Geometry: final body of the model. Coordinates: model frame, mm. A direction names the side the tool comes from. Give positions to 0.01 mm unless a question says otherwise; leave off trailing zeros. Loops run counter-clockwise (first coordinate to the right, second up) from the corner with the lowest first, then second, coordinate; pieces in that order, holes last.
from build123d import *

# Parameters (mm, degrees)
ESQUISSE1_W                          = 200
ESQUISSE1_H                          = 300
BOSS_EXTRU_1_DEPTH                   = 80
COQUE1_T                             = -4
ESQUISSE3_W                          = 196.2
ESQUISSE3_H                          = 296.2
ENL_V_MAT_EXTRU_2_DEPTH              = 4.1
ESQUISSE4_R                          = 9
BOSS_EXTRU_2_DEPTH                   = 67.9
ESQUISSE5_R                          = 2.5
ENL_V_MAT_EXTRU_3_DEPTH              = 30
ESQUISSE4_4_R                        = 9
BOSS_EXTRU_3_DEPTH                   = 15
ESQUISSE6_R                          = 2.5
ENL_V_MAT_EXTRU_6_DEPTH              = 10
ESQUISSE8_R                          = 9
BOSS_EXTRU_5_DEPTH                   = 68
ESQUISSE9_R                          = 2.5
ENL_V_MAT_EXTRU_8_DEPTH              = 30
ESQUISSE10_W                         = 1.9
ESQUISSE10_H                         = 2.840533171
BOSS_EXTRU_6_DEPTH                   = 10
R_P_TITION_LIN_AIRE1_COUNT           = 2
R_P_TITION_LIN_AIRE1_PITCH           = 198.1
R_P_TITION_LIN_AIRE2_COUNT           = 3
R_P_TITION_LIN_AIRE2_PITCH           = 130
R_P_TITION_LIN_AIRE2_COPY_1_SKETCH_W = 1.9
R_P_TITION_LIN_AIRE2_COPY_1_SKETCH_H = 2.840533171
R_P_TITION_LIN_AIRE2_COPY_1_DEPTH    = 10
R_P_TITION_LIN_AIRE2_COPY_2_SKETCH_W = 1.9
R_P_TITION_LIN_AIRE2_COPY_2_SKETCH_H = 2.840533171
R_P_TITION_LIN_AIRE2_COPY_2_DEPTH    = 10


with BuildPart() as part:
    # Esquisse1 → Boss.-Extru.1 (new body)
    with BuildSketch(Plane.XY):
        with Locations((43.373964051, -118.711656442)):
            Rectangle(ESQUISSE1_W, ESQUISSE1_H)
    extrude(amount=BOSS_EXTRU_1_DEPTH)

    # Coque1
    coque1_openings = [part.faces().sort_by_distance(p)[0] for p in [
        (43.373964051, -118.711656442, 0),
    ]]
    offset(amount=COQUE1_T, openings=coque1_openings, kind=Kind.INTERSECTION)

    # Esquisse3 → Enl_v. mat.-Extru.2 (cut)
    with BuildSketch(Plane(origin=(0, 0, 0), x_dir=(-1, 0, 0), z_dir=(0, 0, -1))):
        with Locations((-43.373964051, -118.711656442)):
            Rectangle(ESQUISSE3_W, ESQUISSE3_H)
    extrude(amount=-ENL_V_MAT_EXTRU_2_DEPTH, mode=Mode.SUBTRACT)

    # Esquisse4 → Boss.-Extru.2 (add)
    with BuildSketch(Plane(origin=(0, 0, 76), x_dir=(-1, 0, 0), z_dir=(0, 0, -1))):
        with Locations((-119.373964051, 7.288343558)):
            Circle(ESQUISSE4_R)
    extrude(amount=BOSS_EXTRU_2_DEPTH)

    # Esquisse5 → Enl_v. mat.-Extru.3 (cut)
    with BuildSketch(Plane(origin=(0, 0, 8.1), x_dir=(-1, 0, 0), z_dir=(0, 0, -1))):
        with Locations((-119.373964051, 7.288343558)):
            Circle(ESQUISSE5_R)
    extrude(amount=-ENL_V_MAT_EXTRU_3_DEPTH, mode=Mode.SUBTRACT)

    # Esquisse4_4 → Boss.-Extru.3 (add)
    with BuildSketch(Plane(origin=(0, 0, 76), x_dir=(-1, 0, 0), z_dir=(0, 0, -1))):
        with BuildLine():
            Line((-101.873964051, -42.711656442), (-101.873964051, -51.711656442))
            Line((-101.873964051, -51.711656442), (-110.873964051, -51.711656442))
            ThreePointArc((-110.873964051, -51.711656442), (-101.873964051, -60.711656442), (-92.873964051, -51.711656442))
            ThreePointArc((-92.873964051, -51.711656442), (-95.510003021, -45.347695411), (-101.873964051, -42.711656442))
        make_face()
        with BuildLine():
            Line((-110.873964051, -51.711656442), (-101.873964051, -51.711656442))
            Line((-101.873964051, -51.711656442), (-101.873964051, -42.711656442))
            ThreePointArc((-101.873964051, -42.711656442), (-108.237925082, -45.347695411), (-110.873964051, -51.711656442))
        make_face()
        with BuildLine():
            Line((-101.873964051, -42.711656442), (-101.873964051, -51.711656442))
            Line((-101.873964051, -51.711656442), (-110.873964051, -51.711656442))
            ThreePointArc((-110.873964051, -51.711656442), (-101.873964051, -60.711656442), (-92.873964051, -51.711656442))
            ThreePointArc((-92.873964051, -51.711656442), (-95.510003021, -45.347695411), (-101.873964051, -42.711656442))
        make_face()
        with BuildLine():
            Line((-110.873964051, -51.711656442), (-101.873964051, -51.711656442))
            Line((-101.873964051, -51.711656442), (-101.873964051, -42.711656442))
            ThreePointArc((-101.873964051, -42.711656442), (-108.237925082, -45.347695411), (-110.873964051, -51.711656442))
        make_face()
        with BuildLine():
            Line((15.126035949, -194.711656442), (15.126035949, -185.711656442))
            Line((15.126035949, -185.711656442), (24.126035949, -185.711656442))
            ThreePointArc((24.126035949, -185.711656442), (8.762074918, -179.347695411), (15.126035949, -194.711656442))
        make_face()
        with BuildLine():
            Line((24.126035949, -185.711656442), (15.126035949, -185.711656442))
            Line((15.126035949, -185.711656442), (15.126035949, -194.711656442))
            ThreePointArc((15.126035949, -194.711656442), (21.489996979, -192.075617472), (24.126035949, -185.711656442))
        make_face()
        with BuildLine():
            Line((15.126035949, -194.711656442), (15.126035949, -185.711656442))
            Line((15.126035949, -185.711656442), (24.126035949, -185.711656442))
            ThreePointArc((24.126035949, -185.711656442), (8.762074918, -179.347695411), (15.126035949, -194.711656442))
        make_face()
        with BuildLine():
            Line((24.126035949, -185.711656442), (15.126035949, -185.711656442))
            Line((15.126035949, -185.711656442), (15.126035949, -194.711656442))
            ThreePointArc((15.126035949, -194.711656442), (21.489996979, -192.075617472), (24.126035949, -185.711656442))
        make_face()
        with Locations((15.126035949, -51.711656442)):
            Circle(ESQUISSE4_4_R)
        with Locations((-101.873964051, -185.711656442)):
            Circle(ESQUISSE4_4_R)
    extrude(amount=BOSS_EXTRU_3_DEPTH)

    # Esquisse6 → Enl_v. mat.-Extru.6 (cut)
    with BuildSketch(Plane(origin=(0, 0, 61), x_dir=(-1, 0, 0), z_dir=(0, 0, -1))):
        with Locations((-101.873964051, -51.711656442)):
            Circle(ESQUISSE6_R)
        with Locations((15.126035949, -51.711656442)):
            Circle(ESQUISSE6_R)
        with Locations((-101.873964051, -185.711656442)):
            Circle(ESQUISSE6_R)
        with Locations((15.126035949, -185.711656442)):
            Circle(ESQUISSE6_R)
    extrude(amount=-ENL_V_MAT_EXTRU_6_DEPTH, mode=Mode.SUBTRACT)

    # Esquisse8 → Boss.-Extru.5 (add)
    with BuildSketch(Plane(origin=(0, 0, 76), x_dir=(-1, 0, 0), z_dir=(0, 0, -1))):
        with BuildLine():
            Line((32.626035949, 16.288343558), (32.626035949, 7.288343558))
            Line((32.626035949, 7.288343558), (41.626035949, 7.288343558))
            ThreePointArc((41.626035949, 7.288343558), (38.989996979, 13.652304589), (32.626035949, 16.288343558))
        make_face()
        with BuildLine():
            Line((41.626035949, 7.288343558), (32.626035949, 7.288343558))
            Line((32.626035949, 7.288343558), (32.626035949, 16.288343558))
            ThreePointArc((32.626035949, 16.288343558), (26.262074918, 0.924382528), (41.626035949, 7.288343558))
        make_face()
        with BuildLine():
            Line((32.626035949, 16.288343558), (32.626035949, 7.288343558))
            Line((32.626035949, 7.288343558), (41.626035949, 7.288343558))
            ThreePointArc((41.626035949, 7.288343558), (38.989996979, 13.652304589), (32.626035949, 16.288343558))
        make_face()
        with BuildLine():
            Line((41.626035949, 7.288343558), (32.626035949, 7.288343558))
            Line((32.626035949, 7.288343558), (32.626035949, 16.288343558))
            ThreePointArc((32.626035949, 16.288343558), (26.262074918, 0.924382528), (41.626035949, 7.288343558))
        make_face()
        with BuildLine():
            Line((32.626035949, -253.711656442), (32.626035949, -244.711656442))
            Line((32.626035949, -244.711656442), (41.626035949, -244.711656442))
            ThreePointArc((41.626035949, -244.711656442), (26.262074918, -238.347695411), (32.626035949, -253.711656442))
        make_face()
        with BuildLine():
            Line((41.626035949, -244.711656442), (32.626035949, -244.711656442))
            Line((32.626035949, -244.711656442), (32.626035949, -253.711656442))
            ThreePointArc((32.626035949, -253.711656442), (38.989996979, -251.075617472), (41.626035949, -244.711656442))
        make_face()
        with BuildLine():
            Line((32.626035949, -253.711656442), (32.626035949, -244.711656442))
            Line((32.626035949, -244.711656442), (41.626035949, -244.711656442))
            ThreePointArc((41.626035949, -244.711656442), (26.262074918, -238.347695411), (32.626035949, -253.711656442))
        make_face()
        with BuildLine():
            Line((41.626035949, -244.711656442), (32.626035949, -244.711656442))
            Line((32.626035949, -244.711656442), (32.626035949, -253.711656442))
            ThreePointArc((32.626035949, -253.711656442), (38.989996979, -251.075617472), (41.626035949, -244.711656442))
        make_face()
        with Locations((-119.373964051, -244.711656442)):
            Circle(ESQUISSE8_R)
    extrude(amount=BOSS_EXTRU_5_DEPTH)

    # Esquisse9 → Enl_v. mat.-Extru.8 (cut)
    with BuildSketch(Plane(origin=(0, 0, 8), x_dir=(-1, 0, 0), z_dir=(0, 0, -1))):
        with Locations((32.626035949, 7.288343558)):
            Circle(ESQUISSE9_R)
        with Locations((32.626035949, -244.711656442)):
            Circle(ESQUISSE9_R)
        with Locations((-119.373964051, -244.711656442)):
            Circle(ESQUISSE9_R)
    extrude(amount=-ENL_V_MAT_EXTRU_8_DEPTH, mode=Mode.SUBTRACT)

    # Esquisse10 → Boss.-Extru.6 (add)
    with BuildSketch(Plane(origin=(0, 0, 0), x_dir=(-1, 0, 0), z_dir=(0, 0, -1))):
        with Locations((-142.423964051, -249.983146828)):
            Rectangle(ESQUISSE10_W, ESQUISSE10_H)
    boss_extru_6 = extrude(amount=BOSS_EXTRU_6_DEPTH)

    # R_p_tition lin_aire1: Boss.-Extru.6 ×2
    with Locations(*[(-i * R_P_TITION_LIN_AIRE1_PITCH, 0, 0) for i in range(1, R_P_TITION_LIN_AIRE1_COUNT)]):
        add(boss_extru_6)

    # R_p_tition lin_aire2: Boss.-Extru.6 ×3
    with Locations(*[(0, i * R_P_TITION_LIN_AIRE2_PITCH, 0) for i in range(1, R_P_TITION_LIN_AIRE2_COUNT)]):
        add(boss_extru_6)

    # R_p_tition lin_aire2 copy 1 sketch → R_p_tition lin_aire2 copy 1 (add)
    with BuildSketch(Plane(origin=(-198.1, 130, 0), x_dir=(-1, 0, 0), z_dir=(0, 0, -1))):
        with Locations((-142.423964051, -249.983146828)):
            Rectangle(R_P_TITION_LIN_AIRE2_COPY_1_SKETCH_W, R_P_TITION_LIN_AIRE2_COPY_1_SKETCH_H)
    extrude(amount=R_P_TITION_LIN_AIRE2_COPY_1_DEPTH)

    # R_p_tition lin_aire2 copy 2 sketch → R_p_tition lin_aire2 copy 2 (add)
    with BuildSketch(Plane(origin=(-198.1, 260, 0), x_dir=(-1, 0, 0), z_dir=(0, 0, -1))):
        with Locations((-142.423964051, -249.983146828)):
            Rectangle(R_P_TITION_LIN_AIRE2_COPY_2_SKETCH_W, R_P_TITION_LIN_AIRE2_COPY_2_SKETCH_H)
    extrude(amount=R_P_TITION_LIN_AIRE2_COPY_2_DEPTH)


solid = part.part
Item 1: Section query D-D on x = 35.5. Return loops of the section in (y, z).
Values follow:
outline: (-268.71, 0) - (-266.81, 0) - (-266.81, 4.1) - (-264.71, 4.1) - (-264.71, 76) - (27.29, 76) - (27.29, 4.1) - (29.39, 4.1) - (29.39, 0) - (31.29, 0) - (31.29, 80) - (-268.71, 80) - close
Item 2: Pin query (flat end, axial travel): pin 1 (20 mm diameter, centred on x = -15.5, y = -181.5, fed in from -Z); pin 2 (9 mm diameter, centred on x = -28.5, y = 5, fed in from -Z); pin 3 (19 mm diameter, centred on x = 76.5, y = -264, fed in from -Z). Return the tip coordinate at first contact, or that it passes through.
Values follow:
pin 1: stops at z = 61
pin 2: stops at z = 8
pin 3: stops at z = 0
Item 3: Set-up query: faces 1 (the face through (-52.626, -121, 40)), 2 (the face through (42, -117, 80)). Return all of +Z, -Z, +X, -X, +Y, -Y with unobstructed straight access to the full face (end or side cutting, diameter ignored); none if empty.
Values follow:
face 1: -Z
face 2: +Z, +X, -X, +Y, -Y
Item 4: Section query B-B on z = 22. Give the number of separate pieces and of enclosed holes in the cut face, plus the area to 3 significant figures.
Values follow:
separate pieces: 5
enclosed holes: 5
area: 4,880 mm2
Item 5: Ray query, probe 1 along Y at (x, z) = (135.5, 20); probe 2 along X at (y, z) = (-187, 33); probe 3 along X at (y, z) = (-110, 2). Return the intervals inside material, ascending.
Values follow:
probe 1: y = -268.71 to -264.71, 27.29 to 31.29
probe 2: x = -56.63 to -52.63, 139.37 to 143.37
probe 3: x = -56.63 to -54.73, 141.47 to 143.37
Item 6: Draft query along X for faces 3 (the face through (-56.626, -121, 34)), 4 (the face through (42, 31.288, 39)), 5 (the face through (-19.279, -59.696, 68.605)). Return one class per face: +X half, -X half, draft (parallel to the pull), parting line (faces both ways), or undercut.
Values follow:
face 3: -X half
face 4: draft
face 5: undercut
Item 7: Section query A-A on z = 46. Return loops of the section in (x, y), plus the area to 3 significant figures.
Values follow:
outline: (-56.63, -268.71) - (143.37, -268.71) - (143.37, 31.29) - (-56.63, 31.29) - close; circle Ø18 at (-32.63, -244.71); circle Ø18 at (-32.63, 7.29); circle Ø18 at (119.37, -244.71); circle Ø18 at (119.37, 7.29); hole (-52.63, -264.71) - (139.37, -264.71) - (139.37, 27.29) - (-52.63, 27.29) - close
area: 4,950 mm2
